Verification items for the finished model (mm, model axes). Face numbers are marked on the shaded views. A direction names the side the tool comes from. Round coordinates to 2 decimals unless told otherwise and drop trailing zeros. Write each loop counter-clockwise with the first axis right and the second up, starting at its lowest first coordinate (ties: lowest second). Pieces come first, ordered by that corner, then holes. Notation, with made-up numbers: M 48.5,34 L 61.5,34 A21 ccw 61.5,66 Z; hole C -33.5,71 d9. An arc over 180 degrees is marked long. One line per item, written item: value. Start each with the question number.
Item 1: Tool access check on the marked faces 1 and 2. Record the directions out of +Z, -Z, +X, -X, +Y, -Y that give a thin tool (end or side, any length) a straight path to the whole face; none if there is none.
Item 2: Section check C-C, the plane x = -67. Record the cut outline in (y, z), then the cut area to 3 significant figures.
Item 3: Section check D-D, the plane z = -5. Record the cut outline in (x, y) (3 decimals), then the cut area to 3 significant figures.
Item 4: Section check A-A, the plane y = 0. Record the cut outline in (x, z) (3 decimals), then the cut area to 3 significant figures.
Item 5: Gauge pin test, flat ends, axial feed: pin 1 (1.5 mm diameter, centred on x = -96.5, z = 0, fed in from +Y); pin 2 (6 mm diameter, centred on x = -53, y = 5, fed in from -Z); pin 3 (8 mm diameter, centred on x = -22, y = 3, fed in from +Z). Record the tip position at first contact, or that the pin passes through.
Item 6: Thickness scan on probe 1 along X at (y, z) = (1.5, -5.5) (3 decimals); probe 2 along Y at (x, z) = (-84, 1); probe 3 along Z at (x, y) = (-59, -2). Record the ranges inside material, lowest first. Write a range as from..to.
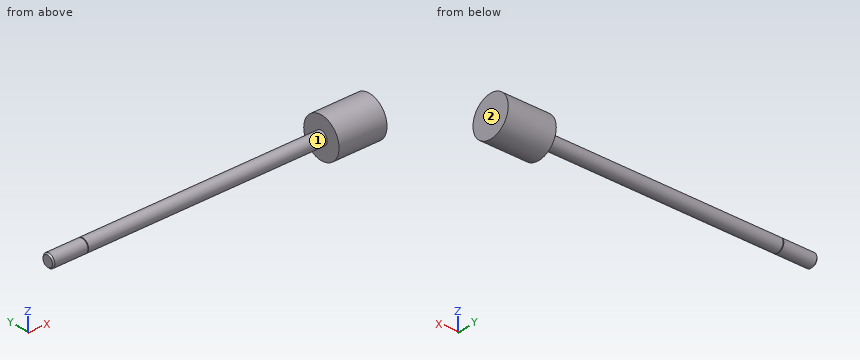
Autodesk Inventor part; units mm, degrees
ref_plane "h1_XY" through (-115.0874, 0, 0) normal (0, 1, 0) x (1, 0, 0)
ref_plane "h1_YZ" through (-115.0874, 0, 0) normal (1, 0, 0) x (0, 0, -1)
ref_plane "h1_ZX" through (-115.0874, 0, 0) normal (0, 0, -1) x (0, 1, 0)
sketch "Sketch_3" plane through (0, 0, 0) normal (0, 0, 1) x (1, 0, 0)
  line L0 (0, 0) -> (-115.0874, 0)
  line L1 (-115.0874, 0) -> (-115.0874, 1.9406)
  line L2 (-115.0874, 1.9406) -> (-114.615, 2.413)
  line L3 (-114.615, 2.413) -> (0, 2.413)
  line L4 (0, 2.413) -> (0, 0)
  line L5 (0, 0) -> (-115.0874, 0)
revolve "Revolution1" add sketch "Sketch_3" angle 360 about axis through (0, 0, 0) along (1, 0, 0)
thread "Thread1"
sketch "Sketch_17" plane through (0, 0, 0) normal (0, 0, 1) x (1, 0, 0)
  line L0 (115.0874, 0) -> (-115.0874, 0)
  line L1 (-102.6414, 2.413) -> (-102.6414, 2.159)
  line L2 (-102.6414, 2.159) -> (-102.3874, 2.159)
  line L3 (-102.3874, 2.159) -> (-102.3874, 2.413)
  line L4 (-102.3874, 2.413) -> (-102.6414, 2.413)
revolve "Revolution2" cut sketch "Sketch_17" angle 360 about axis through (115.0874, 0, 0) along (1, 0, 0)
sketch "Sketch_12" plane through (0, 0, 0) normal (0, 0, 1) x (1, 0, 0)
  line L0 (1.524, 0) -> (-15.875, 0)
  line L1 (-15.875, 0) -> (-15.875, 7.2771)
  line L2 (-15.875, 7.2771) -> (1.524, 7.2771)
  line L3 (1.524, 7.2771) -> (1.524, 0)
  line L4 (1.524, 0) -> (-15.875, 0)
revolve "Revolution3" add sketch "Sketch_12" angle 360 about axis through (1.524, 0, 0) along (1, 0, 0)
ref_plane "h1_XY" through (-115.0874, 0, 0) normal (0, 1, 0) x (1, 0, 0)
ref_plane "h1_YZ" through (-115.0874, 0, 0) normal (1, 0, 0) x (0, 0, -1)
ref_plane "h1_ZX" through (-115.0874, 0, 0) normal (0, 0, -1) x (0, 1, 0)
ref_plane "h2_XY" through (-102.3874, 0, 0) normal (0, 1, 0) x (1, 0, 0)
ref_plane "h2_YZ" through (-102.3874, 0, 0) normal (1, 0, 0) x (0, 0, -1)
ref_plane "h2_ZX" through (-102.3874, 0, 0) normal (0, 0, -1) x (0, 1, 0)
ref_plane "k1_XY" through (-115.0874, 0, -2.413) normal (0, 1, 0) x (1, 0, 0)
ref_plane "k1_YZ" through (-115.0874, 0, -2.413) normal (1, 0, 0) x (0, 0, -1)
ref_plane "k1_ZX" through (-115.0874, 0, -2.413) normal (0, 0, -1) x (0, 1, 0)
ref_plane "k2_XY" through (-115.0874, 0, 2.413) normal (0, 1, 0) x (1, 0, 0)
ref_plane "k2_YZ" through (-115.0874, 0, 2.413) normal (1, 0, 0) x (0, 0, -1)
ref_plane "k2_ZX" through (-115.0874, 0, 2.413) normal (0, 0, -1) x (0, 1, 0)
ref_plane "start_XY" through (-102.3874, 0, 0) normal (0, 1, 0) x (1, 0, 0)
ref_plane "start_YZ" through (-102.3874, 0, 0) normal (1, 0, 0) x (0, 0, -1)
ref_plane "start_ZX" through (-102.3874, 0, 0) normal (0, 0, -1) x (0, 1, 0)
ref_plane "to_prc_XY" through (-102.3874, 0, 0) normal (1, 0, 0) x (0, 0, -1)
ref_plane "to_prc_YZ" through (-102.3874, 0, 0) normal (0, 0, -1) x (0, 1, 0)
ref_plane "to_prc_ZX" through (-102.3874, 0, 0) normal (0, 1, 0) x (1, 0, 0)
ref_plane "to_rod_guide_XY" through (-115.0874, 0, 0) normal (1, 0, 0) x (0, 0, -1)
ref_plane "to_rod_guide_YZ" through (-115.0874, 0, 0) normal (0, 0, -1) x (0, 1, 0)
ref_plane "to_rod_guide_ZX" through (-115.0874, 0, 0) normal (0, 1, 0) x (1, 0, 0)
properties part number "D-75080.25-2XP-4.531-3pos"
Response values:
1. face 1: -X
1. face 2: +Z, -Z, +X, +Y, -Y
2. outline: C 0,0 d4.83
2. area: 18.3 mm2
3. outline: M -15.875,-5.287 L 1.524,-5.287 L 1.524,5.287 L -15.875,5.287 Z
3. area: 184 mm2
4. outline: M -115.087,-1.941 L -114.615,-2.413 L -102.641,-2.413 L -102.641,-2.159 L -102.387,-2.159 L -102.387,-2.413 L -15.875,-2.413 L -15.875,-7.277 L 1.524,-7.277 L 1.524,7.277 L -15.875,7.277 L -15.875,2.413 L -102.387,2.413 L -102.387,2.159 L -102.641,2.159 L -102.641,2.413 L -114.615,2.413 L -115.087,1.941 Z
4. area: 732 mm2
5. pin 1: stops at y = 2.41
5. pin 2: stops at z = -1.35
5. pin 3: stops at z = 2.41
6. probe 1: x = -15.875..1.524
6. probe 2: y = -2.2..2.2
6. probe 3: z = -1.35..1.35
